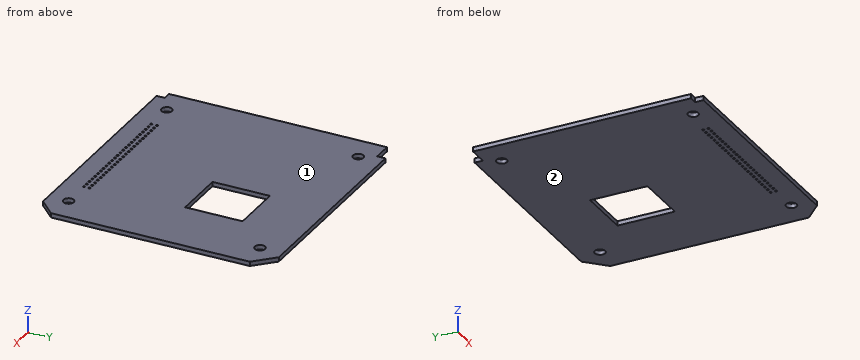
```python
from build123d import *

# Parameters (mm, degrees)
SKETCH1_R           = 1.9
SKETCH1_R_2         = 0.375
BOSS_EXTRUDE1_DEPTH = 1.6
SKETCH_1_W          = 19.5
SKETCH_1_H          = 21
CUT_EXTRUDE_1_DEPTH = 10
SKETCH_2_W          = 7
SKETCH_2_H          = 3
CUT_EXTRUDE_2_DEPTH = 10


with BuildPart() as part:
    # Sketch1 → Boss-Extrude1 (new body)
    with BuildSketch(Plane.XY):
        Polygon((90, -79.7), (90, 0), (0, 0), (0, -82.7), (3, -82.7), (3, -85.7), (84, -85.7), align=None)
        with Locations((10, -78.4)):
            Circle(SKETCH1_R, mode=Mode.SUBTRACT)
        with Locations((10, -8.4)):
            Circle(SKETCH1_R, mode=Mode.SUBTRACT)
        with Locations((80, -8.4)):
            Circle(SKETCH1_R, mode=Mode.SUBTRACT)
        with Locations((80, -78.4)):
            Circle(SKETCH1_R, mode=Mode.SUBTRACT)
        with Locations((21, -76.4)):
            Circle(SKETCH1_R_2, mode=Mode.SUBTRACT)
        with Locations((23, -76.4)):
            Circle(SKETCH1_R_2, mode=Mode.SUBTRACT)
        with Locations((25, -76.4)):
            Circle(SKETCH1_R_2, mode=Mode.SUBTRACT)
        with Locations((27, -76.4)):
            Circle(SKETCH1_R_2, mode=Mode.SUBTRACT)
        with Locations((29, -76.4)):
            Circle(SKETCH1_R_2, mode=Mode.SUBTRACT)
        with Locations((31, -76.4)):
            Circle(SKETCH1_R_2, mode=Mode.SUBTRACT)
        with Locations((33, -76.4)):
            Circle(SKETCH1_R_2, mode=Mode.SUBTRACT)
        with Locations((35, -76.4)):
            Circle(SKETCH1_R_2, mode=Mode.SUBTRACT)
        with Locations((37, -76.4)):
            Circle(SKETCH1_R_2, mode=Mode.SUBTRACT)
        with Locations((39, -76.4)):
            Circle(SKETCH1_R_2, mode=Mode.SUBTRACT)
        with Locations((41, -76.4)):
            Circle(SKETCH1_R_2, mode=Mode.SUBTRACT)
        with Locations((43, -76.4)):
            Circle(SKETCH1_R_2, mode=Mode.SUBTRACT)
        with Locations((45, -76.4)):
            Circle(SKETCH1_R_2, mode=Mode.SUBTRACT)
        with Locations((47, -76.4)):
            Circle(SKETCH1_R_2, mode=Mode.SUBTRACT)
        with Locations((49, -76.4)):
            Circle(SKETCH1_R_2, mode=Mode.SUBTRACT)
        with Locations((51, -76.4)):
            Circle(SKETCH1_R_2, mode=Mode.SUBTRACT)
        with Locations((53, -76.4)):
            Circle(SKETCH1_R_2, mode=Mode.SUBTRACT)
        with Locations((55, -76.4)):
            Circle(SKETCH1_R_2, mode=Mode.SUBTRACT)
        with Locations((57, -76.4)):
            Circle(SKETCH1_R_2, mode=Mode.SUBTRACT)
        with Locations((59, -76.4)):
            Circle(SKETCH1_R_2, mode=Mode.SUBTRACT)
        with Locations((61, -76.4)):
            Circle(SKETCH1_R_2, mode=Mode.SUBTRACT)
        with Locations((63, -76.4)):
            Circle(SKETCH1_R_2, mode=Mode.SUBTRACT)
        with Locations((65, -76.4)):
            Circle(SKETCH1_R_2, mode=Mode.SUBTRACT)
        with Locations((67, -76.4)):
            Circle(SKETCH1_R_2, mode=Mode.SUBTRACT)
        with Locations((69, -76.4)):
            Circle(SKETCH1_R_2, mode=Mode.SUBTRACT)
        with Locations((23, -78.4)):
            Circle(SKETCH1_R_2, mode=Mode.SUBTRACT)
        with Locations((25, -78.4)):
            Circle(SKETCH1_R_2, mode=Mode.SUBTRACT)
        with Locations((27, -78.4)):
            Circle(SKETCH1_R_2, mode=Mode.SUBTRACT)
        with Locations((29, -78.4)):
            Circle(SKETCH1_R_2, mode=Mode.SUBTRACT)
        with Locations((31, -78.4)):
            Circle(SKETCH1_R_2, mode=Mode.SUBTRACT)
        with Locations((33, -78.4)):
            Circle(SKETCH1_R_2, mode=Mode.SUBTRACT)
        with Locations((35, -78.4)):
            Circle(SKETCH1_R_2, mode=Mode.SUBTRACT)
        with Locations((37, -78.4)):
            Circle(SKETCH1_R_2, mode=Mode.SUBTRACT)
        with Locations((39, -78.4)):
            Circle(SKETCH1_R_2, mode=Mode.SUBTRACT)
        with Locations((41, -78.4)):
            Circle(SKETCH1_R_2, mode=Mode.SUBTRACT)
        with Locations((43, -78.4)):
            Circle(SKETCH1_R_2, mode=Mode.SUBTRACT)
        with Locations((45, -78.4)):
            Circle(SKETCH1_R_2, mode=Mode.SUBTRACT)
        with Locations((47, -78.4)):
            Circle(SKETCH1_R_2, mode=Mode.SUBTRACT)
        with Locations((49, -78.4)):
            Circle(SKETCH1_R_2, mode=Mode.SUBTRACT)
        with Locations((51, -78.4)):
            Circle(SKETCH1_R_2, mode=Mode.SUBTRACT)
        with Locations((53, -78.4)):
            Circle(SKETCH1_R_2, mode=Mode.SUBTRACT)
        with Locations((55, -78.4)):
            Circle(SKETCH1_R_2, mode=Mode.SUBTRACT)
        with Locations((57, -78.4)):
            Circle(SKETCH1_R_2, mode=Mode.SUBTRACT)
        with Locations((59, -78.4)):
            Circle(SKETCH1_R_2, mode=Mode.SUBTRACT)
        with Locations((61, -78.4)):
            Circle(SKETCH1_R_2, mode=Mode.SUBTRACT)
        with Locations((63, -78.4)):
            Circle(SKETCH1_R_2, mode=Mode.SUBTRACT)
        with Locations((65, -78.4)):
            Circle(SKETCH1_R_2, mode=Mode.SUBTRACT)
        with Locations((67, -78.4)):
            Circle(SKETCH1_R_2, mode=Mode.SUBTRACT)
        with Locations((69, -78.4)):
            Circle(SKETCH1_R_2, mode=Mode.SUBTRACT)
        with Locations((21, -78.4)):
            Circle(SKETCH1_R_2, mode=Mode.SUBTRACT)
    extrude(amount=BOSS_EXTRUDE1_DEPTH)

    # ｽｹｯﾁ1 → ｶｯﾄ - 押し出し1 (cut)
    with BuildSketch(Plane.XY.offset(1.6)):
        with Locations((56.75, -32.2)):
            Rectangle(SKETCH_1_W, SKETCH_1_H)
    extrude(amount=-CUT_EXTRUDE_1_DEPTH, mode=Mode.SUBTRACT)

    # ｽｹｯﾁ2 → ｶｯﾄ - 押し出し2 (cut)
    with BuildSketch(Plane.XY.offset(1.6)):
        Polygon((90, 0), (90, -7), (83, 0), align=None)
        with Locations((3.5, -1.5)):
            Rectangle(SKETCH_2_W, SKETCH_2_H)
    extrude(amount=-CUT_EXTRUDE_2_DEPTH, mode=Mode.SUBTRACT)


solid = part.part
```
The model under review builds one solid part; all positions refer to its coordinate system, in mm. Face numbers are marked on the shaded views. Coordinates: 2 decimals unless noted, no trailing zeros. Loops run counter-clockwise (first coordinate to the right, second up) from the corner with the lowest first, then second, coordinate; pieces in that order, holes last. Notation, with made-up numbers: (75, 79.25) -> (134, 79.25) arc R21 ccw to (134, 118.25) -> close; hole circle Ø5 at (30, 88.25). An arc over 180 degrees is marked (long way). Answer as CSV lines item,"result".
Item 1: Take a section at B-B, the plane y = -24.5. State the section outline as (x, z) points, and give its area (3 significant figures).
Results below:
outline,"(0, 0) -> (47, 0) -> (47, 1.6) -> (0, 1.6) -> close; (66.5, 0) -> (90, 0) -> (90, 1.6) -> (66.5, 1.6) -> close"
area,"113 mm2"
Item 2: For L1, parallel to Y at x = 25, z = 1.1 (3 decimals); L2, parallel to Y at x = 63, z = 0.9 (3 decimals); L3, parallel to X at y = -7, z = 0.1, list the stretches that pass through material, from the lowest coordinate up.
Results below:
L1,"y = -85.7 to -78.775, -78.025 to -76.775, -76.025 to 0"
L2,"y = -85.7 to -78.775, -78.025 to -76.775, -76.025 to -42.7, -21.7 to 0"
L3,"x = 0 to 8.72, 11.28 to 78.72, 81.28 to 90"
Item 3: Take a section at C-C, the plane z = 0.8. Count the separate pieces of the cut face and the enclosed holes in it, and give its area (3 significant figures).
Results below:
separate pieces,"1"
enclosed holes,"55"
area,"7,160 mm2"
Item 4: Take a section at A-A, the plane x = 10. State the section outline as (y, z) points, and give its area (3 significant figures).
Results below:
outline,"(-85.7, 0) -> (-80.3, 0) -> (-80.3, 1.6) -> (-85.7, 1.6) -> close; (-76.5, 0) -> (-10.3, 0) -> (-10.3, 1.6) -> (-76.5, 1.6) -> close; (-6.5, 0) -> (0, 0) -> (0, 1.6) -> (-6.5, 1.6) -> close"
area,"125 mm2"
Item 5: Draft analysis for pull direction Z (two halves, no side actions). For the marked faces 1 and 2, state which applies: +Z half, -Z half, draft (parallel to the pull), parting line (faces both ways), or undercut.
Results below:
face 1,"+Z half"
face 2,"-Z half"
Item 6: Insertion check: pin 1 (0.5 mm diameter, centred on y = -83.5, z = 1, fed in from -X); pin 2 (0.8 mm diameter, centred on x = 2.5, z = 0.5, fed in from +Y); pin 3 (0.8 mm diameter, centred on x = 1, z = 1, fed in from -Y). Each pin has a flat end and moves straight along its axis. Give the tip position at first contact, or say it passes through.
Results below:
pin 1,"stops at x = 3"
pin 2,"stops at y = -3"
pin 3,"stops at y = -82.7"
